from build123d import *

# Parameters (mm, degrees)
BOSS_EXTRUDE1_DEPTH    = 1.5
SKETCH2_W              = 41
SKETCH2_H              = 40
BOSS_EXTRUDE2_DEPTH    = 1.5
CONVERT_SOLID1_START   = -20
CONVERT_SOLID1_DEPTH   = 40
CONVERT_SOLID1_2_DEPTH = 40
M3_CLEARANCE_HOLE1_D   = 3.2
CIRPATTERN1_COUNT      = 6
CUT_EXTRUDE1_DEPTH     = 54.525694764
M3_CLEARANCE_HOLE2_D   = 3.4
LPATTERN1_COUNT        = 2
LPATTERN1_PITCH        = 24
LPATTERN1_COPY_1_D     = 3.4
FILLET1_R              = 3
CHAMFER1_SIZE          = 0.5
CHAMFER2_SIZE          = 0.5


# Read off the part's stored shape, not the designer's step: Convert-Solid1
with BuildPart() as part:
    # Sketch1 → Boss-Extrude1 (new body)
    with BuildSketch(Plane(origin=(0, 0, 0), x_dir=(0, 0, -1), z_dir=(1, 0, 0))):
        with BuildLine():
            Line((-20, 0), (-20, -28))
            Line((-20, -28), (20, -28))
            Line((20, -28), (20, 0))
            ThreePointArc((20, 0), (0, 20), (-20, 0))
        make_face()
    extrude(amount=BOSS_EXTRUDE1_DEPTH)

    # Sketch2 → Boss-Extrude2 (add)
    with BuildSketch(Plane.XZ.offset(28)):
        with Locations((20.5, 0)):
            Rectangle(SKETCH2_W, SKETCH2_H)
    extrude(amount=-BOSS_EXTRUDE2_DEPTH)

    # Convert-Solid1 outline → Convert-Solid1 (cut)
    with BuildSketch(Plane.XY.offset(CONVERT_SOLID1_START)):
        with BuildLine():
            Line((0, -28), (2.262, -28))
            ThreePointArc((2.262, -28), (0.662524461, -27.337475539), (0, -25.738))
            Line((0, -25.738), (0, -28))
        make_face()
    extrude(amount=CONVERT_SOLID1_DEPTH, mode=Mode.SUBTRACT)

    # Convert-Solid1 2 outline → Convert-Solid1 2 (add)
    with BuildSketch(Plane.XY.offset(CONVERT_SOLID1_START)):
        with BuildLine():
            Line((1.5, -26.5), (2.262, -26.5))
            ThreePointArc((2.262, -26.5), (1.723184633, -26.276815367), (1.5, -25.738))
            Line((1.5, -25.738), (1.5, -26.5))
        make_face()
    extrude(amount=CONVERT_SOLID1_2_DEPTH)

    # M3 Clearance Hole1 (through all)
    with Locations(Plane.ZY):
        with Locations((-15.5, 0)):
            m3_clearance_hole1 = Hole(M3_CLEARANCE_HOLE1_D / 2)

    # CirPattern1: M3 Clearance Hole1 ×6 about axis
    cirpattern1_axis = Axis((0, 0, 0), (1, 0, 0))
    for i in range(1, CIRPATTERN1_COUNT):
        add(m3_clearance_hole1.rotate(cirpattern1_axis, i * 360 / CIRPATTERN1_COUNT), mode=Mode.SUBTRACT)

    # Sketch9 → Cut-Extrude1 (cut, through all)
    with BuildSketch(Plane.ZY):
        with BuildLine():
            Line((6.5, 7), (6.5, -7))
            ThreePointArc((6.5, -7), (0, -13.5), (-6.5, -7))
            Line((-6.5, -7), (-6.5, 7))
            ThreePointArc((-6.5, 7), (0, 13.5), (6.5, 7))
        make_face()
    extrude(amount=-CUT_EXTRUDE1_DEPTH, mode=Mode.SUBTRACT)

    # M3 Clearance Hole2 (through all)
    with Locations(Plane(origin=(0, -26.5, 0), x_dir=(1, 0, 0), z_dir=(0, 1, 0))):
        with Locations((33, 15)):
            m3_clearance_hole2 = Hole(M3_CLEARANCE_HOLE2_D / 2)

    # Mirror1: M3 Clearance Hole2 across plane
    add(m3_clearance_hole2.mirror(Plane.XY), mode=Mode.SUBTRACT)

    # LPattern1: M3 Clearance Hole2 ×2
    with Locations(*[(-i * LPATTERN1_PITCH, 0, 0) for i in range(1, LPATTERN1_COUNT)]):
        add(m3_clearance_hole2, mode=Mode.SUBTRACT)

    # LPattern1 copy 1 (through all)
    with Locations(Plane(origin=(-24, -26.5, 0), x_dir=(1, 0, 0), z_dir=(0, 1, 0))):
        with Locations((33, -15)):
            Hole(LPATTERN1_COPY_1_D / 2)

    # Fillet1
    fillet1_edges = [part.edges().sort_by_distance(p)[0] for p in [
        (41, -27.25, 20),
        (41, -27.25, -20),
    ]]
    fillet(fillet1_edges, radius=FILLET1_R)

    # Chamfer1
    chamfer1_edges = [part.edges().sort_by_distance(p)[0] for p in [
        (0, 12.037753113, -6.95),
    ]]
    chamfer(chamfer1_edges, length=CHAMFER1_SIZE)

    # Chamfer2
    chamfer2_edges = [part.edges().sort_by_distance(p)[0] for p in [
        (0, 0, -13.9),
        (0, 12.037753113, 6.95),
        (0, 0, 13.9),
        (0, -12.037753113, 6.95),
        (0, -12.037753113, -6.95),
    ]]
    chamfer(chamfer2_edges, length=CHAMFER2_SIZE)


solid = part.part
Input: part model. Units: mm. Frame: model coordinates. A direction names the side the tool comes from. Round coordinates to 2 decimals unless told otherwise and drop trailing zeros. Loops run counter-clockwise (first coordinate to the right, second up) from the corner with the lowest first, then second, coordinate; pieces in that order, holes last. Notation, with made-up numbers: (-12.75, 16.25) -> (-2.75, 16.25) arc R12 ccw to (-2.75, 39.25) -> close; hole circle Ø8 at (-11.5, 50). An arc over 180 degrees is marked (long way). Answer as a JSON object with one key per item and string values. Group by question number.
1) Section query B-B on x = 33. Output: boundary loops of the cut face in (y, z).
2) Section query A-A on z = 0. Output: boundary loops of the cut face in (x, y), plus the area to 3 significant figures.
3) Pin query (flat end, axial travel): pin 1 (3 mm diameter, centred on y = 0, z = -15.5, fed in from +X); pin 2 (12 mm diameter, centred on y = -5, z = -9, fed in from +X); pin 3 (1.2 mm diameter, centred on x = 0.5, y = 2.5, fed in from +Z). Return the tip coordinate at first contact, or that it passes through.
4) Section query C-C on y = -3.5. Output: boundary loops of the cut face in (x, z), plus the area to 3 significant figures.
5) Ray query, L1, parallel to Z at x = 9, y = -26.85; L2, parallel to Y at x = 0.9, z = 7.75; L3, parallel to Y at x = 19, z = 5.5. Return the intervals inside material, ascending.
6) Draft query along X for faces 1 (the flat face through (41, -27, 0)), 2 (the cylindrical face through (1, 20, 0)), 3 (the cylindrical face through (10.7, -27.26, 14.93)). Return one class per face: +X half, -X half, draft (parallel to the pull), parting line (faces both ways), or undercut.
7) Section query D-D on x = 14. Output: boundary loops of the cut face in (y, z), plus the area to 3 significant figures.
8) Reachability of faces 4 (the cylindrical face through (31.43, -27.26, -14.35)), 5 (the flat face through (21, -26.5, 0)), 6 (the flat face through (1, 0, -6.5)) from +Z, -Z, +X, -X, +Y, -Y: full face, straight path, thin tool, end or side. Return the list, or none.
Reply:
{
 "1": {"outline": "(-28, -20) -> (-26.5, -20) -> (-26.5, -16.7) -> (-28, -16.7) -> close; (-28, -13.3) -> (-26.5, -13.3) -> (-26.5, 13.3) -> (-28, 13.3) -> close; (-28, 16.7) -> (-26.5, 16.7) -> (-26.5, 20) -> (-28, 20) -> close"},
 "2": {"outline": "(0, -25.74) arc R2.26 ccw to (2.26, -28) -> (41, -28) -> (41, -26.5) -> (2.26, -26.5) arc R0.76 cw to (1.5, -25.74) -> (1.5, -13.5) -> (0, -13.5) -> close; (0, 13.5) -> (1.5, 13.5) -> (1.5, 20) -> (0, 20) -> close", "area": "89.8 mm2"},
 "3": {"pin 1": "passes through", "pin 2": "stops at x = 1.5", "pin 3": "stops at z = 19.91"},
 "4": {"outline": "(0, -20) -> (1.5, -20) -> (1.5, -6.5) -> (0, -6.5) -> close; (0, 6.5) -> (1.5, 6.5) -> (1.5, 20) -> (0, 20) -> close", "area": "40.5 mm2"},
 "5": {"L1": "z = -20 to -16.7, -13.3 to 13.3, 16.7 to 20", "L2": "y = -27.54 to -15.02, -11.82 to 11.82, 15.02 to 18.44", "L3": "y = -28 to -26.5"},
 "6": {"face 1": "+X half", "face 2": "draft", "face 3": "undercut"},
 "7": {"outline": "(-28, -20) -> (-26.5, -20) -> (-26.5, 20) -> (-28, 20) -> close", "area": "60.0 mm2"},
 "8": {"face 4": "+Y, -Y", "face 5": "+Z, -Z, +X, +Y", "face 6": "+X, -X"}
}
